Check sheet for the drawn part. Datum: minimum x, y, z corner. Units: mm. A direction names the side the tool comes from. Give positions to 0.01 mm unless a question says otherwise; leave off trailing zeros. Loops run counter-clockwise (first coordinate to the right, second up) from the corner with the lowest first, then second, coordinate; pieces in that order, holes last. Notation, with made-up numbers: (-5, -20) - (8, -20) arc R35 ccw to (8, 19) - close; hole circle Ø5 at (73, -18). An arc over 180 degrees is marked (long way). Use a Markdown table: item, result. Add a question column.
1. Draft check along X on the marked faces 4, 5 and 6. Enter one of: pulls with the +X half, pulls with the -X half, needs draft (parallel to the pull), parting line crosses it, or undercut.
2. Cross-section at D-D on x = 22.5. Enter the section's corners in (y, z).
3. Depth check by flat-ended pin: P1, Ø1, axis at y = 35.5, z = 2.5, coming from the +X side; P2, Ø1.7, axis at x = 4.4, y = 40, coming from the -Z side; P3, Ø1, axis at x = 31.5, y = 10.5, coming from the -Z side; P4, Ø9, axis at x = 4, y = 24, coming from the -Z side. Enter the tip coordinate at first touch or a pass-through.
4. Set-up check for the marked faces 1, 2 and 3: record each of +Z, -Z, +X, -X, +Y, -Y from which the full face is reachable in a straight line by a thin tool's end or side.
5. Cross-section at B-B on x = 40.6. Enter the section's corners in (y, z), and give its area (3 significant figures).
6. Cross-section at A-A on y = 10. Enter the section's corners in (x, z).
7. Cross-section at C-C on z = 12.5. Enter the section's corners in (x, y).
8. Material ranges on L1, parallel to Y at x = 4.4, z = 8.8; L2, parallel to X at y = 44, z = 14.25 (3 decimals); L3, parallel to Y at x = 41, z = 8.25, recorded low to high.
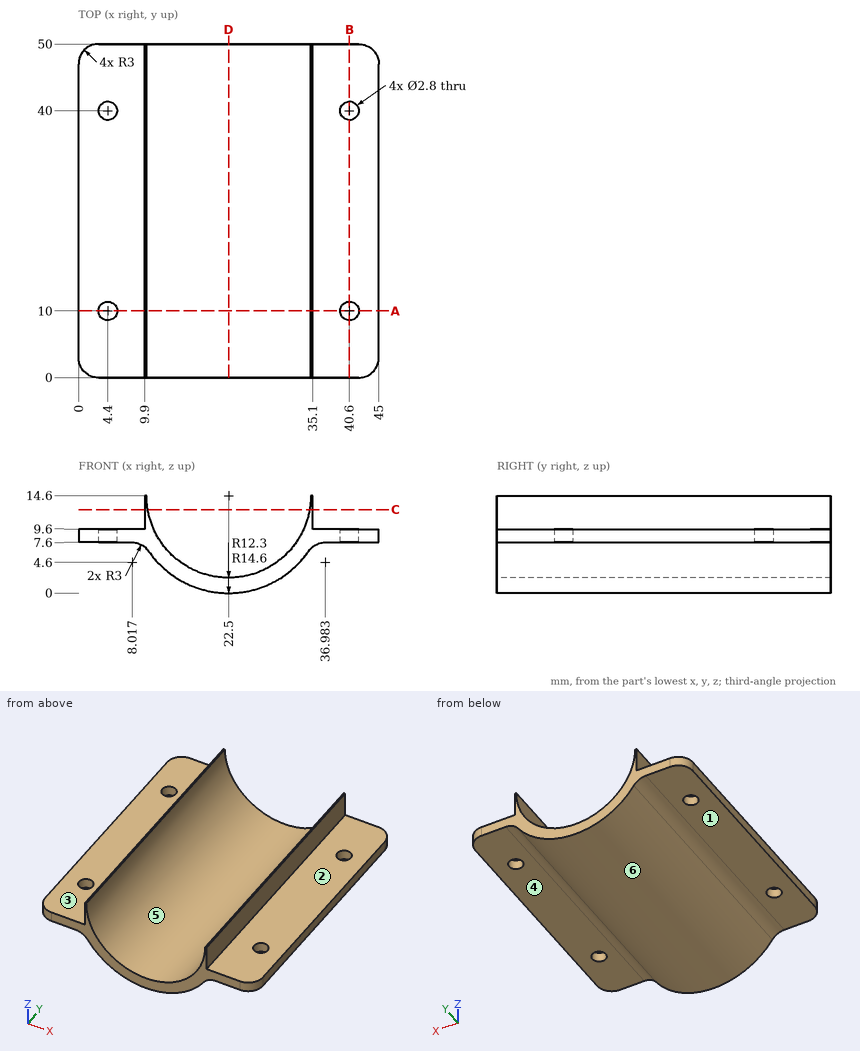
Values found:
| question | item | result |
|---|---|---|
| 1 | face 4 | needs draft |
| 1 | face 5 | undercut |
| 1 | face 6 | parting line crosses it |
| 2 | outline | (0, 0) - (50, 0) - (50, 2.3) - (0, 2.3) - close |
| 3 | P1 | stops at x = 31.37 |
| 3 | P2 | passes through |
| 3 | P3 | stops at z = 2.73 |
| 3 | P4 | stops at z = 7.56 |
| 4 | face 1 | -Z, -X, +Y, -Y |
| 4 | face 2 | +Z, +X, +Y, -Y |
| 4 | face 3 | +Z, -X, +Y, -Y |
| 5 | outline | (0, 7.6) - (8.6, 7.6) - (8.6, 9.6) - (0, 9.6) - close; (11.4, 7.6) - (38.6, 7.6) - (38.6, 9.6) - (11.4, 9.6) - close; (41.4, 7.6) - (50, 7.6) - (50, 9.6) - (41.4, 9.6) - close |
| 5 | area | 88.8 mm2 |
| 6 | outline | (0, 7.6) - (3, 7.6) - (3, 9.6) - (0, 9.6) - close; (5.8, 7.6) - (8.02, 7.6) arc R3 cw to (10.49, 6.3) arc R14.6 ccw to (34.51, 6.3) arc R3 cw to (36.98, 7.6) - (39.2, 7.6) - (39.2, 9.6) - (35.1, 9.6) - (35.1, 14.6) - (34.8, 14.6) arc R12.3 cw to (10.2, 14.6) - (9.9, 14.6) - (9.9, 9.6) - (5.8, 9.6) - close; (42, 7.6) - (45, 7.6) - (45, 9.6) - (42, 9.6) - close |
| 7 | outline | (9.9, 0) - (10.38, 0) - (10.38, 50) - (9.9, 50) - close; (34.62, 0) - (35.1, 0) - (35.1, 50) - (34.62, 50) - close |
| 8 | L1 | y = 0 to 8.6, 11.4 to 38.6, 41.4 to 50 |
| 8 | L2 | x = 9.9 to 10.205, 34.795 to 35.1 |
| 8 | L3 | y = 0 to 8.66, 11.34 to 38.66, 41.34 to 50 |
